Study the drawing (mm; zero at the part's minimum x, y, z) and answer. A direction names the side the tool comes from. Give positions to 0.01 mm unless a question says otherwise; leave off trailing zeros. Loops run counter-clockwise (first coordinate to the right, second up) from the corner with the lowest first, then second, coordinate; pieces in that order, holes last. Notation, with made-up numbers: (80, -21) - (114, -21) arc R22 cw to (114, 10) - close; hole circle Ø6 at (17, 19). An arc over 180 degrees is marked (long way). Use one line per item in the form item = value. Start each with the question number.
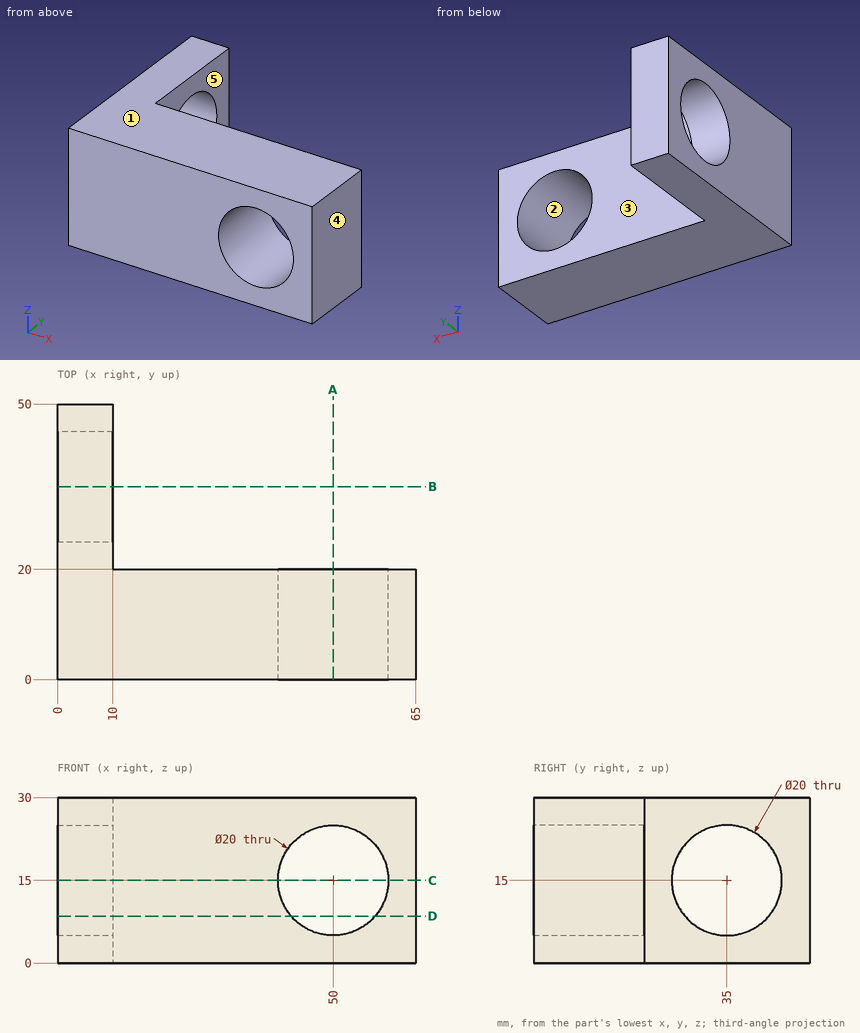
1) A cutting plane is placed at D-D (z = 8.5). Give the vertices of the cut face in (x, y).
2) A cutting plane is placed at B-B (y = 35). Give the vertices of the cut face in (x, z), plus the area to 3 significant figures.
3) A cutting plane is placed at C-C (z = 15). Give the vertices of the cut face in (x, y), plus the area to 3 significant figures.
4) Determine the mould class of the marked faces 1, 2 and 3 for opening direction Z: released by +Z, released by -Z, zero draft, split by the parting line, or undercut.
5) Find the intervals of material crossed by probe 1 along Z at (x, y) = (5.5, 35); probe 2 along X at (y, z) = (12.5, 15); probe 3 along X at (y, z) = (44, 7.25), in increasing order.
6) A cutting plane is placed at A-A (x = 50). Give the vertices of the cut face in (y, z), plus the area to 3 significant figures.
7) A tool of negligible diameter and unlimited length cuts with its end or side. For the marked faces 4 and 5, from which of +Z, -Z, +X, -X, +Y, -Y can it reach the whole face along a straight path? Write none if from no direction.
8) Flat-ended cylindrical pins translate along their axes: pin 1 Ø6 at (x, z) = (22, 20) entering from -Y; pin 2 Ø9 at (x, z) = (26, 21) entering from +Y. Find the tip coordinate at first contact, or state that the pin passes through.
Answer sheet:
q1.outline = (0, 0) - (42.4, 0) - (42.4, 20) - (10, 20) - (10, 27.4) - (0, 27.4) - close; (0, 42.6) - (10, 42.6) - (10, 50) - (0, 50) - close; (57.6, 0) - (65, 0) - (65, 20) - (57.6, 20) - close
q2.outline = (0, 0) - (10, 0) - (10, 5) - (0, 5) - close; (0, 25) - (10, 25) - (10, 30) - (0, 30) - close
q2.area = 100 mm²
q3.outline = (0, 0) - (40, 0) - (40, 20) - (10, 20) - (10, 25) - (0, 25) - close; (0, 45) - (10, 45) - (10, 50) - (0, 50) - close; (60, 0) - (65, 0) - (65, 20) - (60, 20) - close
q3.area = 1,000 mm²
q4.face_1 = released by +Z
q4.face_2 = undercut
q4.face_3 = zero draft
q5.probe_1 = 0 to 5, 25 to 30
q5.probe_2 = 0 to 40, 60 to 65
q5.probe_3 = 0 to 10
q6.outline = (0, 0) - (20, 0) - (20, 5) - (0, 5) - close; (0, 25) - (20, 25) - (20, 30) - (0, 30) - close
q6.area = 200 mm²
q7.face_4 = +Z, -Z, +X, +Y, -Y
q7.face_5 = +Z, -Z, +X, +Y
q8.pin_1 = 0
q8.pin_2 = 20
